Could you check a few things on this model? Use its own coordinates, in mm. Face numbers are marked on the shaded views. Give positions to 0.01 mm unless a question says otherwise; leave off trailing zeros. Write each loop counter-clockwise with the first axis right and the second up, starting at its lowest first coordinate (ties: lowest second). Pieces come first, ordered by that corner, then holes. Notation, with made-up numbers: M 60,62 L 67,62 A18 cw 67,78 Z; hole C 83,28.25 d6. An arc over 180 degrees is marked long. One line per item, written item: value.
```python
from build123d import *

# Parameters (mm, degrees)
CUT_EXTRUDE_541_DEPTH = 1.2
CHAMFER_598_SIZE      = 0.1


with BuildPart() as part:
    # 草图1 → Revolve 358 (revolve)
    with BuildSketch(Plane(origin=(0, 0, 0), x_dir=(1, 0, 0), z_dir=(0, 1, 0)), mode=Mode.PRIVATE) as revolve_358_sk:
        Polygon((0, 0), (0, 3), (1.5, 1.5), (16, 1.5), (16, 0), align=None)
    revolve(revolve_358_sk.sketch.rotate(Axis((0, 0, 0), (1, 0, 0)), 180), axis=Axis((0, 0, 0), (1, 0, 0)))

    # 草图2 → Cut-Extrude 541 (cut)
    with BuildSketch(Plane.ZY):
        Polygon((1.443375673, 0), (0.721687836, 1.25), (-0.721687836, 1.25), (-1.443375673, 0), (-0.721687836, -1.25), (0.721687836, -1.25), align=None)
    extrude(amount=-CUT_EXTRUDE_541_DEPTH, mode=Mode.SUBTRACT)

    # Chamfer 598
    chamfer_598_edges = [part.edges().sort_by_distance(p)[0] for p in [
        (16, 0, -1.5),
    ]]
    chamfer(chamfer_598_edges, length=CHAMFER_598_SIZE)


solid = part.part
```
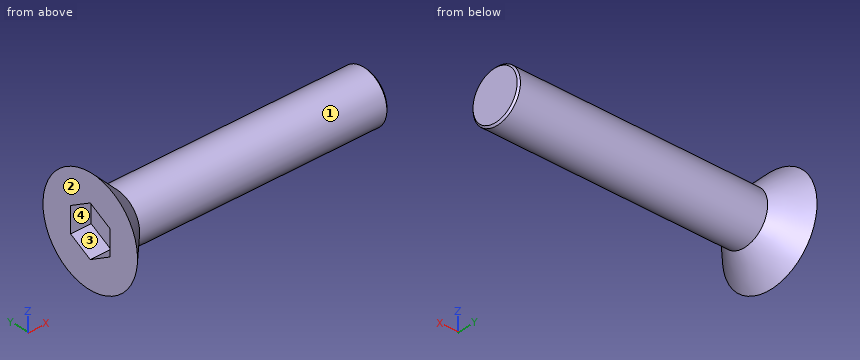
1) If we section it at B-B, the plane x = 7.75: Write out the boundary of the cut face in (y, z), then the cut area to 3 significant figures.
Outcome:
outline: C 0,0 d3
area: 7.07 mm^2
2) We'd pull the mould along Z, two halves only. Please class the marked faces 1, 2, 3 and 4: pulls with the +Z half, pulls with the -Z half, needs draft (parallel to the pull), parting line crosses it, or undercut.
Outcome:
face 1: parting line crosses it
face 2: needs draft
face 3: undercut
face 4: undercut
3) Please list where these lines run through material, in increasing order: L1, parallel to Y at x = 4, z = -0.1; L2, parallel to X at y = -0.2, z = 0.15; L3, parallel to X at y = 1.3, z = 2.2. Write a range as from..to.
Outcome:
L1: y = -1.5..1.5
L2: x = 1.2..16
L3: x = 0..0.44
4) I'm going to push flat-ended pins straight in: pin 1 (2 mm diameter, centred on x = 12, z = 1, fed in from +Y); pin 2 (2 mm diameter, centred on x = 2.5, y = 1, fed in from +Z). Where does each tip first touch, or does it pass through?
Outcome:
pin 1: stops at y = 1.5
pin 2: stops at z = 1.5
5) If we section it at A-A, the plane z = 0: Write out the boundary of the cut face in (x, y).
Outcome:
outline: M 0,-3 L 1.5,-1.5 L 15.9,-1.5 L 16,-1.4 L 16,1.4 L 15.9,1.5 L 1.5,1.5 L 0,3 L 0,1.25 L 1.2,1.25 L 1.2,-1.25 L 0,-1.25 Z
